Design review of the part built by this model. Coordinates are the model's own, in mm. Round coordinates to 2 decimals unless told otherwise and drop trailing zeros. Write each loop counter-clockwise with the first axis right and the second up, starting at its lowest first coordinate (ties: lowest second). Pieces come first, ordered by that corner, then holes. Notation, with made-up numbers: M 72,89.5 L 99,89.5 A18 ccw 99,122.5 Z; hole C 71.5,6.25 d6. An arc over 180 degrees is marked long. Use CSV: the item, a comma, the result in double quotes.
from build123d import *

# Parameters (mm, degrees)
F0_W     = 1351.28
F0_H     = 914.4
F1_DEPTH = 25.4
F3_D     = 12.7
F4_R     = 19.05
F5_DEPTH = 127


with BuildPart() as f1:
    # F0 (on Front) → F1 (new body)
    with BuildSketch(Plane.XZ):
        Rectangle(F0_W, F0_H)
    extrude(amount=F1_DEPTH)

    # F3 (through all)
    with Locations(Plane.XZ.offset(25.4)):
        with Locations((-599.44, -152.4), (-599.44, 0), (-599.44, 152.4), (-599.44, 304.8), (-599.44, -304.8), (599.44, 304.8), (599.44, 152.4), (599.44, 0), (599.44, -152.4), (599.44, -304.8)):
            Hole(F3_D / 2)

    # F4 (on face) → F5 (cut)
    with BuildSketch(Plane.XZ.offset(25.4)):
        with Locations((-311.15, 184.40962)):
            Circle(F4_R)
        with Locations((-311.15, -152.90238)):
            Circle(F4_R)
        with Locations((311.15, -159.049213)):
            Circle(F4_R)
        with Locations((311.15, 178.262787)):
            Circle(F4_R)
    extrude(amount=-F5_DEPTH, mode=Mode.SUBTRACT)


solid = f1.part
1) The part is to be moulded in two halves that separate along X. For faces 1 (the face through (-675.64, -13, -6)), 2 (the face through (-292.98, -12.88, -147.18)), 3 (the face through (675.64, -13, -6)), 4 (the face through (-9, -25.4, 6)), say which applies: released by +X, released by -X, zero draft, split by the parting line, or undercut.
Answers:
face 1,"released by -X"
face 2,"undercut"
face 3,"released by +X"
face 4,"zero draft"
2) Wall thickness on line 1 along Z through (x, y) = (-599.44, -14); line 2 along X through (y, z) = (-16.5, -304.8); line 3 along X through (y, z) = (-7.5, -162): over which ranges is each line inside the solid? List them lowest first. Write a range as [from, to].
Answers:
line 1,"[-457.2, -311.15], [-298.45, -158.75], [-146.05, -6.35], [6.35, 146.05], [158.75, 298.45], [311.15, 457.2]"
line 2,"[-675.64, -605.79], [-593.09, 593.09], [605.79, 675.64]"
line 3,"[-675.64, -327.89], [-294.41, 292.33], [329.97, 675.64]"
3) Add section A-A on x = 311.15. Write out the cut boundary in (y, z), then the cut area to 3 significant figures.
Answers:
outline,"M -25.4,-457.2 L 0,-457.2 L 0,-178.1 L -25.4,-178.1 Z; M -25.4,-140 L 0,-140 L 0,159.21 L -25.4,159.21 Z; M -25.4,197.31 L 0,197.31 L 0,457.2 L -25.4,457.2 Z"
area,"21,300 mm²"
